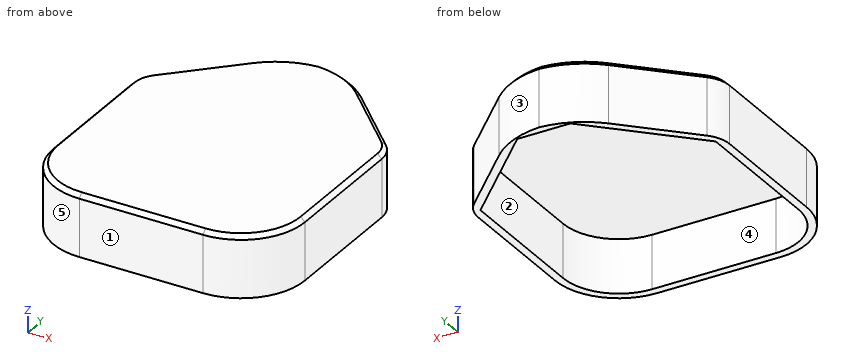
from build123d import *

# Parameters (mm, degrees)
F0_W         = 150
F0_H         = 180.0098
F1_DEPTH     = 36.83
F2_R         = 38.1
F3_R         = 38.1
F4_SIZE      = 57.15
F5_SIZE      = 57.15
F6_T         = -4.826
F7_T1_DEPTH  = 142.0402448428
F8_R         = 19.05
F9_T1_DEPTH  = 51.8894877579
F9_T3_DEPTH  = 76.8690316368
F9_T5_DEPTH  = 73.8
F9_T7_DEPTH  = 51.8894877579
F9_T10_ANGLE = 78.2371868637
F9_T12_ANGLE = 78.2371868637
F9_T14_ANGLE = 45
F9_T16_ANGLE = 90
F9_T18_ANGLE = 90
F9_T20_ANGLE = 45


# Not quite as in the source:
# - a fillet or chamfer that OpenCascade refuses, or shapes differently, is made with other operations: its cross-section is extruded or revolved along the edge and cut away or added


with BuildPart() as f1:
    # F0 (on Top) → F1 (new body)
    with BuildSketch(Plane.XY):
        with Locations((-75, 90.0049)):
            Rectangle(F0_W, F0_H)
    extrude(amount=F1_DEPTH)

    # F2
    f2_edges = [f1.edges().sort_by_distance(p)[0] for p in [
        (0, 0, 18.415),
    ]]
    fillet(f2_edges, radius=F2_R)

    # F3
    f3_edges = [f1.edges().sort_by_distance(p)[0] for p in [
        (-150, 0, 18.415),
    ]]
    fillet(f3_edges, radius=F3_R)

    # F4
    f4_edges = [f1.edges().sort_by_distance(p)[0] for p in [
        (-150, 180.0098, 18.415),
    ]]
    chamfer(f4_edges, length=F4_SIZE)

    # F5
    f5_edges = [f1.edges().sort_by_distance(p)[0] for p in [
        (0, 180.0098, 18.415),
    ]]
    chamfer(f5_edges, length=F5_SIZE)

    # F6
    f6_openings = [f1.faces().sort_by_distance(p)[0] for p in [
        (-75, 82.174731, 0),
    ]]
    offset(amount=F6_T, openings=f6_openings)

    # F7: fillet of radius 50.8 on 2 edges, made by hand

    # F7_s2 → F7_t1 (cut)
    with BuildSketch(Plane.XY.offset(-52.6051224214)):
        with BuildLine():
            ThreePointArc((-71.8079510314, 180.0098), (-91.2482693956, 176.1428802516), (-107.7289755157, 165.1308244843))
            Line((-107.7289755157, 165.1308244843), (-92.85, 180.0098))
            Line((-92.85, 180.0098), (-71.8079510314, 180.0098))
        make_face()
        with BuildLine():
            ThreePointArc((-78.1920489686, 180.0098), (-58.7517306044, 176.1428802516), (-42.2710244843, 165.1308244843))
            Line((-42.2710244843, 165.1308244843), (-57.15, 180.0098))
            Line((-57.15, 180.0098), (-78.1920489686, 180.0098))
        make_face()
    extrude(amount=F7_T1_DEPTH, mode=Mode.SUBTRACT)

    # F8
    f8_edges = [f1.edges().sort_by_distance(p)[0] for p in [
        (-150, 122.8598, 18.415),
        (0, 122.8598, 18.415),
    ]]
    fillet(f8_edges, radius=F8_R)

    # F9: chamfer of 2.54 on 10 edges, made by hand

    # F9_s2 → F9_t1 (cut)
    with BuildSketch(Plane(origin=(-7.9904841816, -7.9904841816, 0), x_dir=(0, 0, 1), z_dir=(0.7071067812, 0.7071067812, 0))):
        Polygon((34.29, -192.9410148932), (36.83, -190.4010148932), (36.83, -192.9410148932), align=None)
    extrude(amount=F9_T1_DEPTH, mode=Mode.SUBTRACT)

    # F9_s4 → F9_t3 (cut)
    with BuildSketch(Plane.XZ.offset(-114.9690316368)):
        Polygon((-150, 34.29), (-147.46, 36.83), (-150, 36.83), align=None)
        Polygon((0, 34.29), (-2.54, 36.83), (0, 36.83), align=None)
    extrude(amount=F9_T3_DEPTH, mode=Mode.SUBTRACT)

    # F9_s6 → F9_t5 (cut)
    with BuildSketch(Plane.YZ.offset(-111.9)):
        Polygon((0, 34.29), (2.54, 36.83), (0, 36.83), align=None)
    extrude(amount=F9_T5_DEPTH, mode=Mode.SUBTRACT)

    # F9_s8 → F9_t7 (cut)
    with BuildSketch(Plane(origin=(-103.7009244843, 103.7009244843, 0), x_dir=(0, 0, 1), z_dir=(0.7071067812, -0.7071067812, 0))):
        Polygon((34.29, -86.8749977152), (36.83, -84.3349977152), (36.83, -86.8749977152), align=None)
    extrude(amount=F9_T7_DEPTH, mode=Mode.SUBTRACT)

    # F9_s9 → F9_t10 (revolve, cut)
    with BuildSketch(Plane(origin=(4.5334842912, 2.9708331336, 0), x_dir=(0, 0, 1), z_dir=(-0.8364087505, -0.548106196, 0))):
        Polygon((34.29, 201.7297538876), (36.83, 199.1897538876), (36.83, 201.7297538876), align=None)
    revolve(axis=Axis((-78.1920489684, 129.2098000003, 36.83), (0, 0, -1)), revolution_arc=F9_T10_ANGLE, mode=Mode.SUBTRACT)

    # F9_s11 → F9_t12 (revolve, cut)
    with BuildSketch(Plane(origin=(28.7009244845, 28.7009244846, 0), x_dir=(0, 0, 1), z_dir=(-0.7071067812, -0.7071067812, 0))):
        Polygon((34.29, 192.9410148931), (36.83, 190.4010148931), (36.83, 192.9410148931), align=None)
    revolve(axis=Axis((-71.8079510316, 129.2098000003, 36.83), (0, 0, -1)), revolution_arc=F9_T12_ANGLE, mode=Mode.SUBTRACT)

    # F9_s13 → F9_t14 (revolve, cut)
    with BuildSketch(Plane.XZ.offset(-114.9690316368)):
        Polygon((-150, 34.29), (-147.46, 36.83), (-150, 36.83), align=None)
    revolve(axis=Axis((-130.95, 114.9690316368, 36.83), (0, 0, -1)), revolution_arc=F9_T14_ANGLE, mode=Mode.SUBTRACT)

    # F9_s15 → F9_t16 (revolve, cut)
    with BuildSketch(Plane.YZ.offset(-111.9)):
        Polygon((0, 34.29), (2.54, 36.83), (0, 36.83), align=None)
    revolve(axis=Axis((-111.9, 38.1, 36.83), (0, 0, -1)), revolution_arc=F9_T16_ANGLE, mode=Mode.SUBTRACT)

    # F9_s17 → F9_t18 (revolve, cut)
    with BuildSketch(Plane.YZ.offset(-38.1)):
        Polygon((0, 34.29), (2.54, 36.83), (0, 36.83), align=None)
    revolve(axis=Axis((-38.1, 38.1, 36.83), (0, 0, 1)), revolution_arc=F9_T18_ANGLE, mode=Mode.SUBTRACT)

    # F9_s19 → F9_t20 (revolve, cut)
    with BuildSketch(Plane(origin=(-67.0095158184, 67.0095158184, 0), x_dir=(0, 0, 1), z_dir=(-0.7071067812, 0.7071067812, 0))):
        Polygon((34.29, 86.8749977152), (36.83, 84.3349977152), (36.83, 86.8749977152), align=None)
    revolve(axis=Axis((-19.05, 114.9690316368, 36.83), (0, 0, -1)), revolution_arc=F9_T20_ANGLE, mode=Mode.SUBTRACT)


solid = f1.part
Input: part model. Units: mm. Frame: model coordinates. Face numbers are marked on the shaded views. A direction names the side the tool comes from. Coordinates: 2 decimals unless noted, no trailing zeros. Loops run counter-clockwise (first coordinate to the right, second up) from the corner with the lowest first, then second, coordinate; pieces in that order, holes last.
Q1. Draft query along Y for the marked faces 3, 4 and 5. Return one class per face: +Y half, -Y half, draft (parallel to the pull), parting line (faces both ways), or undercut.
Q2. Contact query for flat-ended pins moving along their axis: pin 1 (12 mm diameter, centred on x = -16, z = 26, fed in from -Y); pin 2 (10 mm diameter, centred on x = -92, y = 138, fed in from -Z); pin 3 (6 mm diameter, centred on y = 128.5, z = 12.5, fed in from +X). Output: stop coordinate, or through.
Q3. Cut plane B-B (y = 61.5). Output: boundary loops of the cut face in (x, z), then the cut area to 3 significant figures.
Q4. Set-up query: the marked faces 1 and 2. Return all of +Z, -Z, +X, -X, +Y, -Y with unobstructed straight access to the full face (end or side cutting, diameter ignored); none if empty.
Q5. Material intervals for line 1 (Y direction, x = -88, z = 8); line 2 (X direction, y = 39.5, z = 17.5); line 3 (X direction, y = 144.5, z = 26), sorted ascending.
Q6. Cut plane C-C (y = 145). Output: boundary loops of the cut face in (x, z).
Q7. Cut plane A-A (z = 24). Output: boundary loops of the cut face in (x, y).
Working result:
1. face 3: +Y half
1. face 4: undercut
1. face 5: -Y half
2. pin 1: stops at y = 3.57
2. pin 2: stops at z = 32
2. pin 3: stops at x = -3.18
3. outline: (-150, 0) - (-145.17, 0) - (-145.17, 32) - (-4.83, 32) - (-4.83, 0) - (0, 0) - (0, 34.29) - (-2.54, 36.83) - (-147.46, 36.83) - (-150, 34.29) - close
3. area: 1,030 mm2
4. face 1: +Z, -Z, +X, -X, -Y
4. face 2: -Z
5. line 1: y = 0 to 4.83, 175.18 to 177.36
5. line 2: x = -150 to -145.17, -4.83 to 0
5. line 3: x = -128.36 to -121.53, -28.47 to -21.64
6. outline: (-127.86, 0) - (-121.03, 0) - (-121.03, 32) - (-28.97, 32) - (-28.97, 0) - (-22.14, 0) - (-22.14, 34.29) - (-25.73, 36.83) - (-124.27, 36.83) - (-127.86, 34.29) - close
7. outline: (-150, 38.1) arc R38.1 ccw to (-111.9, 0) - (-38.1, 0) arc R38.1 ccw to (0, 38.1) - (0, 114.97) arc R19.05 ccw to (-5.58, 128.44) - (-42.27, 165.13) arc R50.8 ccw to (-75, 179.91) arc R50.8 ccw to (-107.73, 165.13) - (-144.42, 128.44) arc R19.05 ccw to (-150, 114.97) - close; hole (-145.17, 38.1) arc R33.27 ccw to (-111.9, 4.83) - (-38.1, 4.83) arc R33.27 ccw to (-4.83, 38.1) - (-4.83, 120.86) - (-59.15, 175.18) - (-90.85, 175.18) - (-145.17, 120.86) - close
